Here's how the part is built. I have some questions about the finished solid (model axes, mm). Coordinates: 2 decimals unless noted, no trailing zeros. Order: outer loops, then holes, each group sorted by start corner. A loop starts at its lowest first (then second) coordinate and runs counter-clockwise, first axis right, second up. Notation, with made-up numbers: (-5, 71) - (34, 71) arc R14 ccw to (34, 89) - close; hole circle Ø8 at (19.25, 33). An arc over 180 degrees is marked (long way). Answer as CSV lines item,"result". Start each with the question number.
Q1. I need wall thicknesses on line 1 (Y direction, x = -2, z = 8.25); line 2 (X direction, y = 5.5, z = 15); line 3 (X direction, y = 5, z = 20). Which ranges of each line are inside material? Lowest first, please.
Q2. Suppose I cut it at B-B (y = 8). Please give me the cut outline in (x, z).
Q3. For pin 1 Ø1 at (x, z) = (-3.5, 3) entering from -Y; pin 2 Ø6 at (x, z) = (-6.5, 13.5) entering from +Y; pin 3 Ø8 at (y, z) = (5, 16.5) entering from +X, each with a flat end and sliding along its axis, tell me the tip position at first contact or that it passes through.
Q4. Suppose I cut it at A-A (z = 17.5). Please give me the cut outline in (x, y).
Q5. Suppose I cut it at C-C (x = 1). Please give me the cut outline in (y, z), then the cut area to 3 significant figures.
Q6. Suppose I cut it at D-D (x = -13). Please give me the cut outline in (y, z), then the cut area to 3 significant figures.
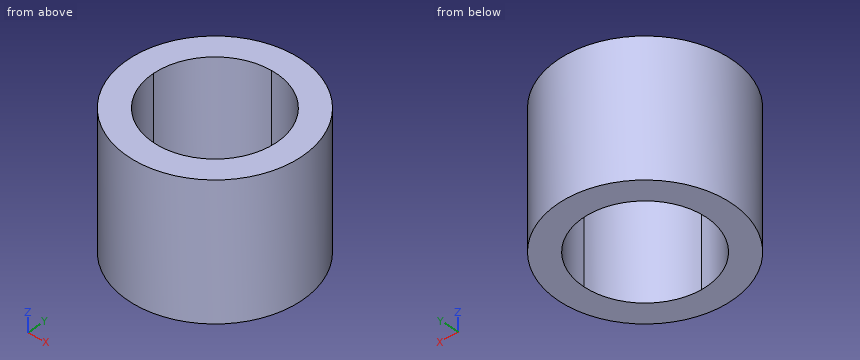
from build123d import *

# Parameters (mm, degrees)
F0_R     = 15.5
F1_DEPTH = 24


with BuildPart() as f1:
    # F0 (on Top) → F1 (new body)
    with BuildSketch(Plane.XY):
        Circle(F0_R)
        with BuildLine():
            ThreePointArc((0, 11.75), (8.3085046789, 8.3085046789), (11.75, 0))
            ThreePointArc((11.75, 0), (8.3085046789, -8.3085046789), (0, -11.75))
            ThreePointArc((0, -11.75), (-8.3085046789, -8.3085046789), (-11.75, 0))
            ThreePointArc((-11.75, 0), (-8.3085046789, 8.3085046789), (0, 11.75))
        make_face(mode=Mode.SUBTRACT)
        with BuildLine():
            ThreePointArc((0, 11), (7.7781745931, 7.7781745931), (11, 0))
            Line((11, 0), (11.75, 0))
            ThreePointArc((11.75, 0), (8.3085046789, 8.3085046789), (0, 11.75))
            Line((0, 11.75), (0, 11))
        make_face()
        with BuildLine():
            ThreePointArc((-11, 0), (-7.7781745931, 7.7781745931), (0, 11))
            Line((0, 11), (0, 11.75))
            ThreePointArc((0, 11.75), (-8.3085046789, 8.3085046789), (-11.75, 0))
            Line((-11.75, 0), (-11, 0))
        make_face()
        with BuildLine():
            Line((0, -11.75), (0, -11))
            ThreePointArc((0, -11), (-7.7781745931, -7.7781745931), (-11, 0))
            Line((-11, 0), (-11.75, 0))
            ThreePointArc((-11.75, 0), (-8.3085046789, -8.3085046789), (0, -11.75))
        make_face()
        with BuildLine():
            Line((11.75, 0), (11, 0))
            ThreePointArc((11, 0), (7.7781745931, -7.7781745931), (0, -11))
            Line((0, -11), (0, -11.75))
            ThreePointArc((0, -11.75), (8.3085046789, -8.3085046789), (11.75, 0))
        make_face()
    extrude(amount=F1_DEPTH)


solid = f1.part
Here are the results:
1,line 1,"y = -15.37 to -10.82, 10.82 to 15.37"
1,line 2,"x = -14.49 to -9.53, 9.53 to 14.49"
1,line 3,"x = -14.67 to -9.8, 9.8 to 14.67"
2,outline,"(-13.28, 0) - (-7.55, 0) - (-7.55, 24) - (-13.28, 24) - close; (7.55, 0) - (13.28, 0) - (13.28, 24) - (7.55, 24) - close"
3,pin 1,"stops at y = -15.21"
3,pin 2,"stops at y = 15.1"
3,pin 3,"stops at x = 15.47"
4,outline,"circle Ø31 at (0, 0); hole circle Ø22 at (0, 0)"
5,outline,"(-15.47, 0) - (-10.95, 0) - (-10.95, 24) - (-15.47, 24) - close; (10.95, 0) - (15.47, 0) - (15.47, 24) - (10.95, 24) - close"
5,area,"217 mm²"
6,outline,"(-8.44, 0) - (8.44, 0) - (8.44, 24) - (-8.44, 24) - close"
6,area,"405 mm²"
